```python
from build123d import *

# Parameters (mm, degrees)
F0_R     = 25.4
F1_DEPTH = 5.08
F2_R     = 3.81
F0_R_2   = 3.302
F3_DEPTH = 5.08


with BuildPart() as f1:
    # F0 (on Front) → F1 (new body, symmetric)
    with BuildSketch(Plane.XZ):
        Circle(F0_R)
        with BuildLine():
            ThreePointArc((18.9545106806, 1.9049999628), (19.0261126937, 0.9536958462), (19.05, 0))
            ThreePointArc((19.05, 0), (19.0261128131, -0.9536934636), (18.9545111577, -1.9049952154))
            ThreePointArc((18.9545111577, -1.9049952154), (17.5999062473, -7.2901166031), (14.749902222, -12.0558236733))
            ThreePointArc((14.749902222, -12.0558236733), (13.4703854002, -13.4703829631), (12.0558263419, -14.7499000408))
            ThreePointArc((12.0558263419, -14.7499000408), (7.2901213153, -17.5999042954), (1.905001936, -18.9545104823))
            ThreePointArc((1.905001936, -18.9545104823), (1.3528e-06, -19.05), (-1.904999244, -18.9545107529))
            ThreePointArc((-1.904999244, -18.9545107529), (-7.2901189565, -17.5999052725), (-12.055824483, -14.7499015601))
            ThreePointArc((-12.055824483, -14.7499015601), (-13.4703841719, -13.4703841913), (-14.7499015428, -12.0558245042))
            ThreePointArc((-14.7499015428, -12.0558245042), (-17.5999039961, -7.2901220379), (-18.9545100886, -1.9050058538))
            ThreePointArc((-18.9545100886, -1.9050058538), (-19.05, -2.3188e-06), (-18.9545105523, 1.9050012395))
            ThreePointArc((-18.9545105523, 1.9050012395), (-17.5999046178, 7.290120537), (-14.7499006641, 12.0558255794))
            ThreePointArc((-14.7499006641, 12.0558255794), (-13.4703834119, 13.4703849513), (-12.0558238937, 14.7499020418))
            ThreePointArc((-12.0558238937, 14.7499020418), (-7.2901186049, 17.5999054181), (-1.904999244, 18.9545107529))
            ThreePointArc((-1.904999244, 18.9545107529), (-2.13e-07, 19.05), (1.9049988201, 18.9545107955))
            ThreePointArc((1.9049988201, 18.9545107955), (7.2901186408, 17.5999054032), (12.0558242838, 14.749901723))
            ThreePointArc((12.0558242838, 14.749901723), (13.4703837424, 13.4703846208), (14.7499009369, 12.0558252456))
            ThreePointArc((14.7499009369, 12.0558252456), (17.5999049458, 7.2901197452), (18.9545106806, 1.9049999628))
        make_face(mode=Mode.SUBTRACT)
    extrude(amount=F1_DEPTH, both=True)

    # F2
    f2_edges = [f1.edges().sort_by_distance(p)[0] for p in [
        (-25.4, 5.08, 0),
        (-25.4, -5.08, 0),
    ]]
    fillet(f2_edges, radius=F2_R)

    # F0 (on Front) → F3 (join, symmetric)
    with BuildSketch(Plane.XZ):
        with BuildLine():
            ThreePointArc((18.9545111577, -1.9049952154), (19.0261128131, -0.9536934636), (19.05, 0))
            ThreePointArc((19.05, 0), (19.0261126937, 0.9536958462), (18.9545106806, 1.9049999628))
            Line((18.9545106806, 1.9049999628), (4.5990766623, 1.9050004462))
            Line((4.5990766623, 1.9050004462), (14.7499009369, 12.0558252456))
            ThreePointArc((14.7499009369, 12.0558252456), (13.4703837424, 13.4703846208), (12.0558242838, 14.749901723))
            Line((12.0558242838, 14.749901723), (1.905, 4.5990772875))
            Line((1.905, 4.5990772875), (1.9049988201, 18.9545107955))
            ThreePointArc((1.9049988201, 18.9545107955), (-2.13e-07, 19.05), (-1.904999244, 18.9545107529))
            Line((-1.904999244, 18.9545107529), (-1.904999244, 4.5990775438))
            Line((-1.904999244, 4.5990775438), (-12.0558238937, 14.7499020418))
            ThreePointArc((-12.0558238937, 14.7499020418), (-13.4703834119, 13.4703849513), (-14.7499006641, 12.0558255794))
            Line((-14.7499006641, 12.0558255794), (-4.599075316, 1.905000756))
            Line((-4.599075316, 1.905000756), (-18.9545105523, 1.9050012395))
            ThreePointArc((-18.9545105523, 1.9050012395), (-19.05, -2.3188e-06), (-18.9545100886, -1.9050058538))
            Line((-18.9545100886, -1.9050058538), (-4.5990790156, -1.9050018252))
            Line((-4.5990790156, -1.9050018252), (-14.7499015428, -12.0558245042))
            ThreePointArc((-14.7499015428, -12.0558245042), (-13.4703841719, -13.4703841913), (-12.055824483, -14.7499015601))
            Line((-12.055824483, -14.7499015601), (-1.904999244, -4.5990757963))
            Line((-1.904999244, -4.5990757963), (-1.904999244, -18.9545107529))
            ThreePointArc((-1.904999244, -18.9545107529), (1.3528e-06, -19.05), (1.905001936, -18.9545104823))
            Line((1.905001936, -18.9545104823), (1.905000756, -4.5990749797))
            Line((1.905000756, -4.5990749797), (12.0558263419, -14.7499000408))
            ThreePointArc((12.0558263419, -14.7499000408), (13.4703854002, -13.4703829631), (14.749902222, -12.0558236733))
            Line((14.749902222, -12.0558236733), (4.599077641, -1.904999244))
            Line((4.599077641, -1.904999244), (18.9545111577, -1.9049952154))
        make_face()
        Circle(F0_R_2, mode=Mode.SUBTRACT)
    extrude(amount=F3_DEPTH, both=True)


solid = f1.part
```
Read the model definition and answer for the solid it produces. Units are mm, in the model's axes. Give positions to 0.01 mm unless a question says otherwise; leave off trailing zeros. Write each loop counter-clockwise with the first axis right and the second up, starting at its lowest first coordinate (ties: lowest second). Pieces come first, ordered by that corner, then holes. Notation, with made-up numbers: (66.25, 13) -> (97.25, 13) arc R29 ccw to (97.25, 48) -> close; hole circle Ø11 at (19.25, 60). An arc over 180 degrees is marked (long way). Answer in a Markdown table with one row per item.
1) Section C-C on x = 0 is taken. Give the vertices of the cut face in (y, z).
Results list:
| item | result |
|---|---|
| outline | (-5.08, -21.59) arc R3.81 ccw to (-1.27, -25.4) -> (1.27, -25.4) arc R3.81 ccw to (5.08, -21.59) -> (5.08, -3.3) -> (-5.08, -3.3) -> close; (-5.08, 3.3) -> (5.08, 3.3) -> (5.08, 21.59) arc R3.81 ccw to (1.27, 25.4) -> (-1.27, 25.4) arc R3.81 ccw to (-5.08, 21.59) -> close |
2) Straight lines are drawn through the part: line 1 (Z direction, x = -3, y = 4.5); line 2 (X direction, y = -3, z = -13) (3 decimals); line 3 (X direction, y = 3, z = 2). For each, find the intervals that lie inside material, in ascending order. Write a range as [from, to].
Results list:
| item | result |
|---|---|
| line 1 | [-23.42, -18.81], [-5.69, -1.38], [1.38, 5.69], [18.81, 23.42] |
| line 2 | [-21.336, -10.306], [-1.905, 1.905], [10.306, 21.336] |
| line 3 | [-24.9, -18.94], [-4.69, -2.63], [2.63, 4.69], [18.94, 24.9] |
3) Section A-A on z = 0 is taken. Give the vertices of the cut face in (x, y).
Results list:
| item | result |
|---|---|
| outline | (-25.4, -1.27) arc R3.81 ccw to (-21.59, -5.08) -> (-3.3, -5.08) -> (-3.3, 5.08) -> (-21.59, 5.08) arc R3.81 ccw to (-25.4, 1.27) -> close; (3.3, -5.08) -> (21.59, -5.08) arc R3.81 ccw to (25.4, -1.27) -> (25.4, 1.27) arc R3.81 ccw to (21.59, 5.08) -> (3.3, 5.08) -> close |
4) Each of these flat-tipped pins is pushed along its axis until it touches: pin 1 Ø1.5 at (x, y) = (-15.5, 1) entering from +Z; pin 2 Ø2 at (y, z) = (-0.5, -10) entering from +X; pin 3 Ø2 at (x, z) = (14, -8.5) entering from +Y; pin 4 Ø3 at (y, z) = (1, -12) entering from -X. Where does it stop, or does it pass through?
Results list:
| item | result |
|---|---|
| pin 1 | z = 20.68 |
| pin 2 | x = 23.75 |
| pin 3 | through |
| pin 4 | x = -23.13 |
5) Determine the mould class of faces 1 (the flat face through (4, -5.08, 0)), 2 (the cylindrical face through (-5.506, -0.018, -24.796)), 3 (the flat face through (12, 0, -1.905)) for opening direction Z: released by +Z, released by -Z, zero draft, split by the parting line, or undercut.
Results list:
| item | result |
|---|---|
| face 1 | zero draft |
| face 2 | split by the parting line |
| face 3 | undercut |
6) Section B-B on y = 0 is taken. Count the separate pieces of the cut face and the enclosed holes in it, plus the area to 3 significant figures.
Results list:
| item | result |
|---|---|
| separate pieces | 1 |
| enclosed holes | 9 |
| area | 1,360 mm^2 |
